Input: part model. Units: mm. Frame: model coordinates. A direction names the side the tool comes from. Give positions to 0.01 mm unless a question says otherwise; leave off trailing zeros. Order: outer loops, then holes, each group sorted by start corner. A loop starts at its lowest first (then second) coordinate and runs counter-clockwise, first axis right, second up. Notation, with made-up numbers: (46.5, -13) - (61.5, -13) arc R24 cw to (61.5, 26) - close; hole circle Ø8 at (12, -38). An arc over 180 degrees is marked (long way). Use a Markdown table: item, result.
from build123d import *

# Parameters (mm, degrees)
F0_R     = 85
F0_R_2   = 2.5
F0_R_3   = 6
F1_DEPTH = 5
F0_R_4   = 90
F2_DEPTH = 18
F3_DEPTH = 10


with BuildPart() as f1:
    # F0 (on Front) → F1 (new body)
    with BuildSketch(Plane.XZ):
        with Locations((0.529671, -0.305805)):
            Circle(F0_R)
        with Locations((-12.990381, -7.5)):
            Circle(F0_R_2, mode=Mode.SUBTRACT)
        with Locations((12.990381, -7.5)):
            Circle(F0_R_2, mode=Mode.SUBTRACT)
        with Locations((-40, 35.5)):
            Circle(F0_R_2, mode=Mode.SUBTRACT)
        Circle(F0_R_3, mode=Mode.SUBTRACT)
        with Locations((0, 15)):
            Circle(F0_R_2, mode=Mode.SUBTRACT)
        with Locations((40, 35.5)):
            Circle(F0_R_2, mode=Mode.SUBTRACT)
        with Locations((0, 75.5)):
            Circle(F0_R_2, mode=Mode.SUBTRACT)
    extrude(amount=F1_DEPTH)

    # F0 (on Front) → F2 (join)
    with BuildSketch(Plane.XZ):
        Circle(F0_R_4)
        with Locations((0.529671, -0.305805)):
            Circle(F0_R, mode=Mode.SUBTRACT)
    extrude(amount=F2_DEPTH)

    # F0 (on Front) → F3 (join)
    with BuildSketch(Plane.XZ):
        with Locations((0.529671, -0.305805)):
            Circle(F0_R)
        with Locations((-12.990381, -7.5)):
            Circle(F0_R_2, mode=Mode.SUBTRACT)
        with Locations((12.990381, -7.5)):
            Circle(F0_R_2, mode=Mode.SUBTRACT)
        with Locations((-40, 35.5)):
            Circle(F0_R_2, mode=Mode.SUBTRACT)
        Circle(F0_R_3, mode=Mode.SUBTRACT)
        with Locations((0, 15)):
            Circle(F0_R_2, mode=Mode.SUBTRACT)
        with Locations((40, 35.5)):
            Circle(F0_R_2, mode=Mode.SUBTRACT)
        with Locations((0, 75.5)):
            Circle(F0_R_2, mode=Mode.SUBTRACT)
    extrude(amount=F3_DEPTH)


solid = f1.part
1. Section query D-D (z = 75.5). Return loops of the section in (x, y).
Response:
| item | result |
|---|---|
| outline | (-48.99, -18) - (-37.92, -18) - (-37.92, -10) - (-2.5, -10) - (-2.5, 0) - (-48.99, 0) - close; (2.5, -10) - (38.98, -10) - (38.98, -18) - (48.99, -18) - (48.99, 0) - (2.5, 0) - close |
2. Section query A-A (x = -40). Return loops of the section in (y, z).
Response:
| item | result |
|---|---|
| outline | (-18, -80.62) - (0, -80.62) - (0, 33) - (-10, 33) - (-10, -75.02) - (-18, -75.02) - close; (-18, 74.41) - (-10, 74.41) - (-10, 38) - (0, 38) - (0, 80.62) - (-18, 80.62) - close |
3. Set-up query: faces 4 (the face through (-1, -10, -18)), 5 (the face through (-37.69, -4.93, 34.54)). Return all of +Z, -Z, +X, -X, +Y, -Y with unobstructed straight access to the full face (end or side cutting, diameter ignored); none if empty.
Response:
| item | result |
|---|---|
| face 4 | -Y |
| face 5 | +Y, -Y |
4. Material intervals for line 1 along Z through (x, y) = (0, -2.75); line 2 along X through (y, z) = (-1.5, -7); line 3 along Y through (x, z) = (3.5, 22), sorted ascending.
Response:
| item | result |
|---|---|
| line 1 | z = -90 to -6, 6 to 12.5, 17.5 to 73, 78 to 90 |
| line 2 | x = -89.73 to -15.44, -10.54 to 10.54, 15.44 to 89.73 |
| line 3 | y = -10 to 0 |
5. Section query B-B (y = -5.25). Return loops of the section in (x, z).
Response:
| item | result |
|---|---|
| outline | circle Ø180 at (0, 0); hole circle Ø5 at (-40, 35.5); hole circle Ø5 at (-12.99, -7.5); hole circle Ø12 at (0, 0); hole circle Ø5 at (0, 15); hole circle Ø5 at (0, 75.5); hole circle Ø5 at (12.99, -7.5); hole circle Ø5 at (40, 35.5) |
6. Pin query (flat end, axial travel): pin 1 (1.5 mm diameter, centred on x = -9, y = -8.5, fed in from +Z); pin 2 (5 mm diameter, centred on y = -4.5, z = 36, fed in from -X); pin 3 (6 mm diameter, centred on y = -8.5, z = 4, fed in from -X). Return the tip coordinate at first contact, or that it passes through.
Response:
| item | result |
|---|---|
| pin 1 | stops at z = 89.62 |
| pin 2 | stops at x = -83.53 |
| pin 3 | stops at x = -89.99 |
7. Mould query, pull axis X, two halves, no side actions, for faces 1 (the face through (-10.7, -4.9, -8.5)), 2 (the face through (41.53, -8.874, -79.845)), 3 (the face through (-80.4, -18, 27.1)). Classes: pulls with the +X half, pulls with the -X half, needs draft (parallel to the pull), parting line crosses it, or undercut.
Response:
| item | result |
|---|---|
| face 1 | undercut |
| face 2 | parting line crosses it |
| face 3 | needs draft |
8. Section query C-C (x = 0). Return loops of the section in (y, z), then the cut area to 3 significant figures.
Response:
| item | result |
|---|---|
| outline | (-18, -90) - (0, -90) - (0, -6) - (-10, -6) - (-10, -85.3) - (-18, -85.3) - close; (-18, 84.69) - (-10, 84.69) - (-10, 78) - (0, 78) - (0, 90) - (-18, 90) - close; (-10, 6) - (0, 6) - (0, 12.5) - (-10, 12.5) - close; (-10, 17.5) - (0, 17.5) - (0, 73) - (-10, 73) - close |
| area | 1,660 mm^2 |
